The listing builds one solid part. Answer for the finished solid, in the listing's coordinates (mm). Face numbers are marked on the shaded views. A direction names the side the tool comes from. Give positions to 0.01 mm unless a question says otherwise; leave off trailing zeros. Write each loop counter-clockwise with the first axis right and the second up, starting at its lowest first coordinate (ties: lowest second). Pieces come first, ordered by that corner, then holes. Notation, with made-up numbers: (2, -17.5) -> (25, -17.5) arc R23 ccw to (25, -8.5) -> close; hole circle Ø11 at (-19, 39.25). An arc over 180 degrees is marked (long way). One line per question, with ' | ' between items.
from build123d import *

# Parameters (mm, degrees)
F0_R     = 4
F0_W     = 35
F0_H     = 35
F0_R_2   = 1.5
F0_R_3   = 11.1
F1_DEPTH = 4
F2_DEPTH = 40
F4_DEPTH = 96.501
F5_R     = 5
F7_DEPTH = 44.001
F9_DEPTH = 44.001
F10_R    = 5


with BuildPart() as f1:
    # F0 (on Right) → F1 (new body)
    with BuildSketch(Plane.YZ):
        Polygon((-51.5, 80.5), (-89.5, 80.5), (-89.5, -7), (7, -7), (7, 0), align=None)
        with Locations((-84, 0)):
            Circle(F0_R, mode=Mode.SUBTRACT)
        Circle(F0_R, mode=Mode.SUBTRACT)
        with Locations((-69, 60)):
            Rectangle(F0_W, F0_H, mode=Mode.SUBTRACT)
        with Locations((-69, 60)):
            Rectangle(F0_W, F0_H)
        with Locations((-81.8535834551, 46.8301847577)):
            Circle(F0_R_2, mode=Mode.SUBTRACT)
        with Locations((-56, 47)):
            Circle(F0_R_2, mode=Mode.SUBTRACT)
        with Locations((-69, 60)):
            Circle(F0_R_3, mode=Mode.SUBTRACT)
        with Locations((-82, 73)):
            Circle(F0_R_2, mode=Mode.SUBTRACT)
        with Locations((-55.9914708138, 72.9807242751)):
            Circle(F0_R_2, mode=Mode.SUBTRACT)
    extrude(amount=F1_DEPTH)

    # F0 (on Right) → F2 (join)
    with BuildSketch(Plane.YZ):
        Polygon((-51.5, 80.5), (-89.5, 80.5), (-89.5, -7), (7, -7), (7, 0), align=None)
        with Locations((-84, 0)):
            Circle(F0_R, mode=Mode.SUBTRACT)
        Circle(F0_R, mode=Mode.SUBTRACT)
        with Locations((-69, 60)):
            Rectangle(F0_W, F0_H, mode=Mode.SUBTRACT)
    extrude(amount=-F2_DEPTH)

    # F3 (on face) → F4 (cut, through all)
    with BuildSketch(Plane.XZ.offset(89.5)):
        Polygon((-40, 7), (0, 80.5), (-40, 80.5), align=None)
    extrude(amount=-F4_DEPTH, mode=Mode.SUBTRACT)

    # F5
    f5_edges = [f1.edges().sort_by_distance(p)[0] for p in [
        (-18, -89.5, -7),
        (-18, 7, -7),
        (-18, 7, 0),
        (2, -89.5, 80.5),
        (2, -51.5, 80.5),
    ]]
    fillet(f5_edges, radius=F5_R)

    # F6 (on face) → F7 (cut, through all)
    with BuildSketch(Plane.YZ.offset(4)):
        Polygon((-23.8850931677, 42.5), (-50.0025195443, 78.4393645012), (-50.0025195443, 42.5), align=None)
    extrude(amount=-F7_DEPTH, mode=Mode.SUBTRACT)

    # F8 (on face) → F9 (cut, through all)
    with BuildSketch(Plane.YZ.offset(4)):
        Polygon((0, 9.6324786325), (-23.8850931677, 42.5), (-50.0025195443, 42.5), align=None)
    extrude(amount=-F9_DEPTH, mode=Mode.SUBTRACT)

    # F10
    f10_edges = [f1.edges().sort_by_distance(p)[0] for p in [
        (-8.340136, -50.00252, 42.5),
        (-17.283679, 0, 9.632479),
    ]]
    fillet(f10_edges, radius=F10_R)


solid = f1.part
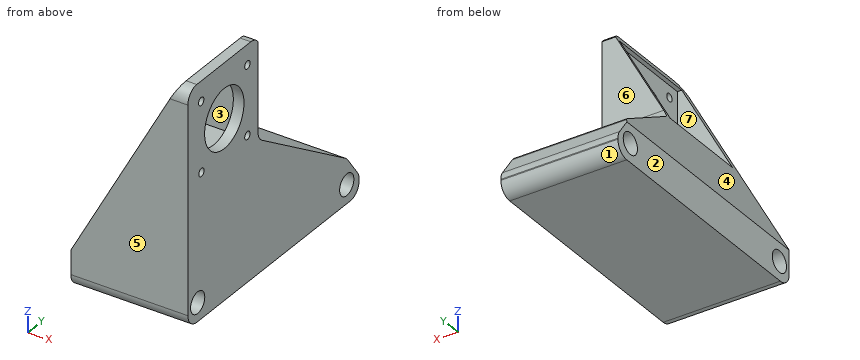
Item 1: Flat-ended cylindrical pins translate along their axes: pin 1 (3.5 mm diameter, centred on y = -82, z = 73, fed in from -X); pin 2 (6 mm diameter, centred on x = -11, y = -72.5, fed in from +Z); pin 3 (1.5 mm diameter, centred on x = -30.5, z = 21.5, fed in from +Y). Find the tip coordinate at first contact, or state that the pin passes through.
Answers below:
pin 1: x = 0 | pin 2: z = 42.5 | pin 3: y = -16.91
Item 2: Find section A-A (y = -69). Write down the section's boundary in (x, z), then the cut area to 3 significant figures.
Answers below:
outline: (-40, -7) -> (4, -7) -> (4, 48.9) -> (0, 48.9) -> (0, 42.5) -> (-20.68, 42.5) -> (-40, 7) -> close; (-1.63, 77.5) -> (0, 77.5) -> (0, 71.1) -> (4, 71.1) -> (4, 80.5) -> (0, 80.5) -> close | area: 1,900 mm²
Item 3: Find section B-B (z = 60). Write down the section's boundary in (x, y).
Answers below:
outline: (-11.16, -89.5) -> (4, -89.5) -> (4, -80.1) -> (0, -80.1) -> (0, -86.5) -> (-11.16, -86.5) -> close; (-11.16, -51.5) -> (0, -51.5) -> (0, -57.9) -> (4, -57.9) -> (4, -50) -> (-11.16, -50) -> close
Item 4: Find section D-D (x = -34.5). Write down the section's boundary in (y, z), then the cut area to 3 significant figures.
Answers below:
outline: (-89.5, -2) arc R5 ccw to (-84.5, -7) -> (2, -7) arc R5 ccw to (7, -2) -> (7, -1.62) arc R5 ccw to (6.04, 1.31) -> (0.54, 8.89) arc R5 ccw to (-0.76, 10.13) -> (-11.37, 17.11) -> (-89.5, 17.11) -> close; hole circle Ø8 at (-84, 0); hole circle Ø8 at (0, 0) | area: 2,090 mm²
Item 5: A tool of negligible diameter and unlimited length cuts with its end or side. For the marked faces 5, 6 and 7, from which of +Z, -Z, +X, -X, +Y, -Y can it reach the whole face along a straight path? Write none if from no direction.
Answers below:
face 5: +Z, -Z, +X, -X, -Y | face 6: +Z, +X, -X, +Y | face 7: -X
Item 6: Determine the mould class of the marked faces 1, 2, 3 and 4 for opening direction Z: pulls with the +Z half, pulls with the -Z half, needs draft (parallel to the pull), parting line crosses it, or undercut.
Answers below:
face 1: pulls with the -Z half | face 2: needs draft | face 3: undercut | face 4: pulls with the +Z half
Item 7: Find section C-C (y = -82). Write down the section's boundary in (x, z).
Answers below:
outline: (-40, -7) -> (4, -7) -> (4, -3.46) -> (-40, -3.46) -> close; (-40, 3.46) -> (4, 3.46) -> (4, 45.34) -> (0, 45.34) -> (0, 42.5) -> (-20.68, 42.5) -> (-40, 7) -> close; (-1.63, 77.5) -> (0, 77.5) -> (0, 74.5) -> (4, 74.5) -> (4, 80.5) -> (0, 80.5) -> close; (0, 48.32) -> (4, 48.32) -> (4, 71.5) -> (0, 71.5) -> close
Item 8: Consider line 1 (Y direction, x = 3, z = 73); line 2 (Y direction, x = -10, z = -1.5); line 3 (Z direction, x = 3.05, y = -69). Determine where each line is inside the solid, lowest interval first. Write a range as [from, to].
Answers below:
line 1: [-89.5, -83.5], [-80.5, -57.49], [-54.49, -50] | line 2: [-89.5, -87.71], [-80.29, -3.71], [3.71, 7] | line 3: [-7, 48.9], [71.1, 80.5]
